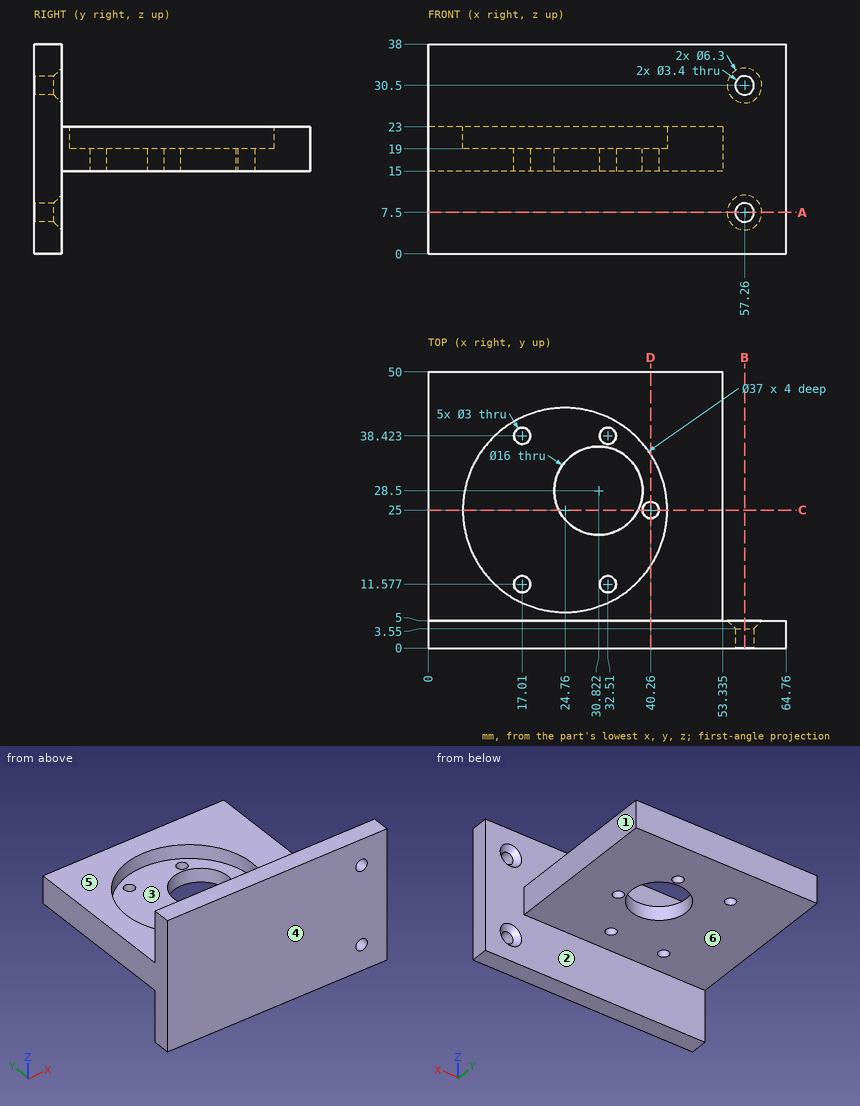
Design review of the part shown in the three views and the two pictorial views. Dimensions are in mm from the part's minimum x, y and z. A direction names the side the tool comes from. Coordinates: 2 decimals unless noted, no trailing zeros. Write each loop counter-clockwise with the first axis right and the second up, starting at its lowest first coordinate (ties: lowest second). Pieces come first, ordered by that corner, then holes.
1) We need section C-C on y = 25. State the section outline as (x, z) points (1 decimal), then the cut area to 3 significant figures.
2) We need section A-A on z = 7.5. State the section outline as (x, y) points.
3) The part is to be moulded in two halves that separate along X. For the marked faces 1, 2 and 3, say which applies: pulls with the +X half, pulls with the -X half, needs draft (parallel to the pull), parting line crosses it, or undercut.
4) To check wall thickness, follow probe 1 along Y at (x, z) = (17.01, 16.9); probe 2 along Y at (x, z) = (24.76, 21.65); probe 3 along Z at (x, y) = (57, 2). State the ranges of each line that lie inside material, in increasing order.
5) We need section D-D on x = 40.26. State the section outline as (y, z) points, then the cut area to 3 significant figures.
6) Clearance check with flat-ended pins moving along their axes: pin 1 Ø1.8 at (x, y) = (32.51, 38.42) entering from -Z; pin 2 Ø2 at (x, z) = (41.5, 7.5) entering from +Y; pin 3 Ø5 at (x, y) = (17.01, 11.58) entering from -Z; pin 4 Ø4 at (y, z) = (26.5, 21) entering from +X (3 decimals). State where each tip first meets the part, or that it passes through.
7) Machinability: for the marked faces 4, 5 and 6, which of the approach directions +Z, -Z, +X, -X, +Y, -Y give a long, thin tool a straight path to every point of the face, cutting with its end or side? Answer none if there is none.
8) We need section B-B on x = 57.26. State the section outline as (y, z) points.
Answer list:
1. outline: (0, 15) - (23.6, 15) - (23.6, 19) - (6.3, 19) - (6.3, 23) - (0, 23) - close; (38, 15) - (38.8, 15) - (38.8, 19) - (38, 19) - close; (41.8, 15) - (53.3, 15) - (53.3, 23) - (43.3, 23) - (43.3, 19) - (41.8, 19) - close
1. area: 209 mm2
2. outline: (0, 0) - (55.56, 0) - (55.56, 3.55) - (54.11, 5) - (0, 5) - close; (58.96, 0) - (64.76, 0) - (64.76, 5) - (60.41, 5) - (58.96, 3.55) - close
3. face 1: pulls with the +X half
3. face 2: needs draft
3. face 3: undercut
4. probe 1: y = 0 to 10.08, 13.08 to 36.92, 39.92 to 50
4. probe 2: y = 0 to 6.5, 43.5 to 50
4. probe 3: z = 0 to 5.82, 9.18 to 28.82, 32.18 to 38
5. outline: (0, 0) - (5, 0) - (5, 15) - (23.5, 15) - (23.5, 19) - (14.9, 19) - (14.9, 23) - (5, 23) - (5, 38) - (0, 38) - close; (26.5, 15) - (50, 15) - (50, 23) - (35.1, 23) - (35.1, 19) - (26.5, 19) - close
5. area: 457 mm2
6. pin 1: passes through
6. pin 2: stops at y = 5
6. pin 3: stops at z = 15
6. pin 4: stops at x = 53.335
7. face 4: +Z, -Z, +X, -X, -Y
7. face 5: +Z, +X, -X, +Y
7. face 6: -Z, +X, -X, +Y
8. outline: (0, 0) - (5, 0) - (5, 4.35) - (3.55, 5.8) - (0, 5.8) - close; (0, 9.2) - (3.55, 9.2) - (5, 10.65) - (5, 27.35) - (3.55, 28.8) - (0, 28.8) - close; (0, 32.2) - (3.55, 32.2) - (5, 33.65) - (5, 38) - (0, 38) - close
